Could you check a few things on this drawing? It's one solid part, dimensions in mm from its lowest x, y, z. A direction names the side the tool comes from. Round coordinates to 2 decimals unless told otherwise and drop trailing zeros. Write each loop counter-clockwise with the first axis right and the second up, starting at its lowest first coordinate (ties: lowest second). Pieces come first, ordered by that corner, then holes. Notation, with made-up numbers: (-11.75, 53) -> (30.25, 53) arc R25 cw to (30.25, 92) -> close; hole circle Ø11 at (29, -28.5). An arc over 180 degrees is marked (long way). Answer in a Markdown table with one row per item.
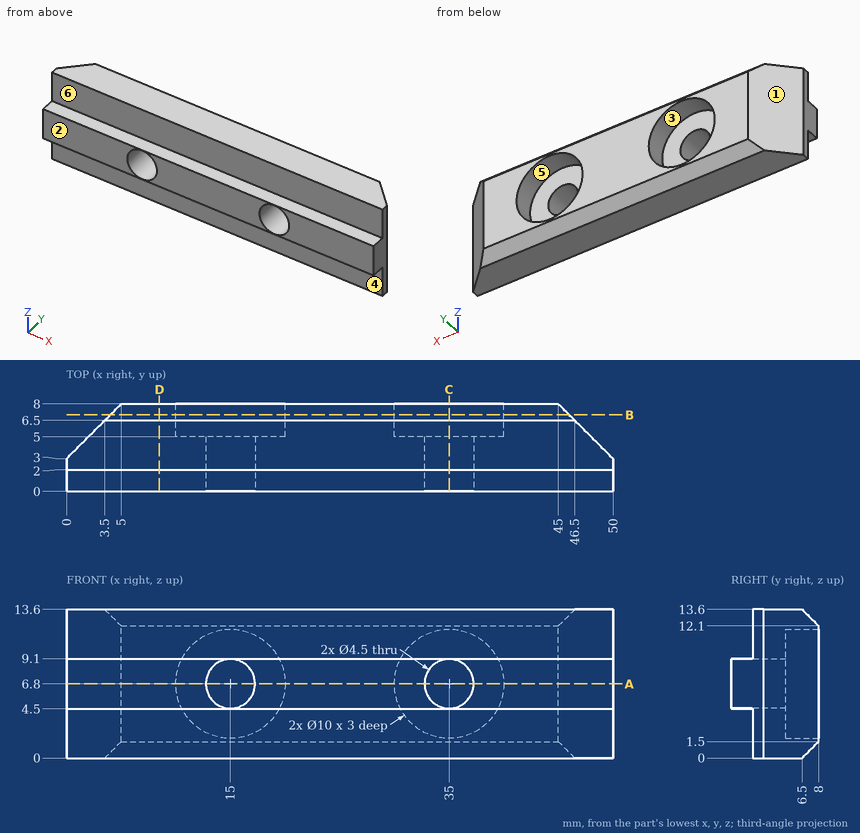
1) I want a section at D-D, the plane x = 8.5. List the corners of the cut face in (y, z) for me, and give its area (4 significant figures).
Response:
| item | result |
|---|---|
| outline | (0, 4.5) -> (2, 4.5) -> (2, 0) -> (6.5, 0) -> (8, 1.5) -> (8, 12.1) -> (6.5, 13.6) -> (2, 13.6) -> (2, 9.1) -> (0, 9.1) -> close |
| area | 88.55 mm^2 |
2) We'd pull the mould along X, two halves only. Please class the marked faces 1, 2 and 3: +X half, -X half, draft (parallel to the pull), parting line (faces both ways), or undercut.
Response:
| item | result |
|---|---|
| face 1 | -X half |
| face 2 | draft |
| face 3 | undercut |
3) I want a section at A-A, the plane z = 6.8. List the corners of the cut face in (x, y) for me.
Response:
| item | result |
|---|---|
| outline | (0, 0) -> (12.75, 0) -> (12.75, 5) -> (10, 5) -> (10, 8) -> (5, 8) -> (0, 3) -> close; (17.25, 0) -> (32.75, 0) -> (32.75, 5) -> (30, 5) -> (30, 8) -> (20, 8) -> (20, 5) -> (17.25, 5) -> close; (37.25, 0) -> (50, 0) -> (50, 3) -> (45, 8) -> (40, 8) -> (40, 5) -> (37.25, 5) -> close |
4) I want a section at B-B, the plane y = 7. List the corners of the cut face in (x, z) for me.
Response:
| item | result |
|---|---|
| outline | (4, 0.5) -> (46, 0.5) -> (46, 13.1) -> (4, 13.1) -> close; hole circle Ø10 at (15, 6.8); hole circle Ø10 at (35, 6.8) |
5) For pin 1 (4 mm diameter, centred on y = 6.5, z = 1.5, fed in from -X); pin 2 (1.5 mm diameter, centred on y = 5.5, z = 4, fed in from +X); pin 3 (6 mm diameter, centred on x = 35, z = 6.8, fed in from +Y), each with a flat end and sliding along its axis, tell me the tip position at first contact or that it passes through.
Response:
| item | result |
|---|---|
| pin 1 | stops at x = 1.5 |
| pin 2 | stops at x = 48.25 |
| pin 3 | stops at y = 5 |
6) I need wall thicknesses on line 1 (Z direction, x = 15, y = 3.6); line 2 (Z direction, x = 35, y = 5.6); line 3 (X direction, y = 7.25, z = 11.25). Which ranges of each line are inside material? Lowest first, please. Write a range as [from, to].
Response:
| item | result |
|---|---|
| line 1 | z = [0, 4.55], [9.05, 13.6] |
| line 2 | z = [0, 1.8], [11.8, 13.6] |
| line 3 | x = [4.25, 12.72], [17.28, 32.72], [37.28, 45.75] |
7) I want a section at C-C, the plane x = 35. List the corners of the cut face in (y, z) for me, and give its area (4 significant figures).
Response:
| item | result |
|---|---|
| outline | (0, 4.5) -> (2, 4.5) -> (2, 0) -> (6.5, 0) -> (8, 1.5) -> (8, 1.8) -> (5, 1.8) -> (5, 4.55) -> (0, 4.55) -> close; (0, 9.05) -> (5, 9.05) -> (5, 11.8) -> (8, 11.8) -> (8, 12.1) -> (6.5, 13.6) -> (2, 13.6) -> (2, 9.1) -> (0, 9.1) -> close |
| area | 36.05 mm^2 |
8) Which directions (+Z, -Z, +X, -X, +Y, -Y) give clear straight access to the entire face, cutting with the end or side of a thin tool? Please do the marked faces 4, 5 and 6.
Response:
| item | result |
|---|---|
| face 4 | -Z, +X, -X, -Y |
| face 5 | +Y |
| face 6 | +Z, +X, -X, -Y |
